The model under review builds one solid part; all positions refer to its coordinate system, in mm. A direction names the side the tool comes from. Round coordinates to 2 decimals unless told otherwise and drop trailing zeros. Write each loop counter-clockwise with the first axis right and the second up, starting at its lowest first coordinate (ties: lowest second). Pieces come first, ordered by that corner, then holes.
Item 1: Add section C-C (z = -13). Give the boundary of the cut face in (x, y), plus the area to 3 significant figures.
Item 2: Add section B-B (x = 4.75). Give the boundary of the cut face in (y, z), plus the area to 3 significant figures.
Item 3: Draft analysis for pull direction Y (two halves, no side actions). For faces 1 (the face through (0, 0, -45)), 2 (the face through (19, 0, -23)), state which applies: +Y half, -Y half, draft (parallel to the pull), parting line (faces both ways), or undercut.
Item 4: Add section A-A (y = 0). Give the boundary of the cut face in (x, z).
Item 5: To check wall thickness, follow L1, parallel to Z at x = 11, y = 0.4; L2, parallel to Z at x = 4.5, y = 0.15; L3, parallel to X at y = 0.7, z = -2. State the ranges of each line that lie inside material, in increasing order.
Item 6: Machinability: for faces 3 (the face through (7, 0, -44)), 4 (the face through (0, 0, 0)), which of the approach directions +Z, -Z, +X, -X, +Y, -Y give a long, thin tool a straight path to every point of the face, cutting with its end or side? Answer none if there is none.
```python
from build123d import *

# Parameters (mm, degrees)
SKETCH_1_R = 1


with BuildPart() as part:
    # По траектории1: sweep along a curve in space
    with BuildLine() as sweep_1_path:
        Line((0, 0, 0), (15, 0, 0))
        ThreePointArc((15, 0, 0), (17.121320344, 0, -0.878679656), (18, 0, -3))
        Line((18, 0, -3), (18, 0, -42))
        ThreePointArc((18, 0, -42), (17.121320344, 0, -44.121320344), (15, 0, -45))
        Line((15, 0, -45), (0, 0, -45))
    # Эскиз1 → По траектории1 (sweep)
    with BuildSketch(Plane(origin=(0, 0, 0), x_dir=(0, 0, -1), z_dir=(1, 0, 0))):
        Circle(SKETCH_1_R)
    sweep(path=sweep_1_path.line)


solid = part.part
```
Numbers:
1. outline: circle Ø2 at (18, 0)
1. area: 3.14 mm2
2. outline: circle Ø2 at (0, -45); circle Ø2 at (0, 0)
2. area: 6.28 mm2
3. face 1: draft
3. face 2: parting line
4. outline: (0, -46) - (15, -46) arc R4 ccw to (19, -42) - (19, -3) arc R4 ccw to (15, 1) - (0, 1) - (0, -1) - (15, -1) arc R2 cw to (17, -3) - (17, -42) arc R2 cw to (15, -44) - (0, -44) - close
5. L1: z = -45.92 to -44.08, -0.92 to 0.92
5. L2: z = -45.99 to -44.01, -0.99 to 0.99
5. L3: x = 17.06 to 18.58
6. face 3: -X
6. face 4: +Z, -Z, -X, +Y, -Y
